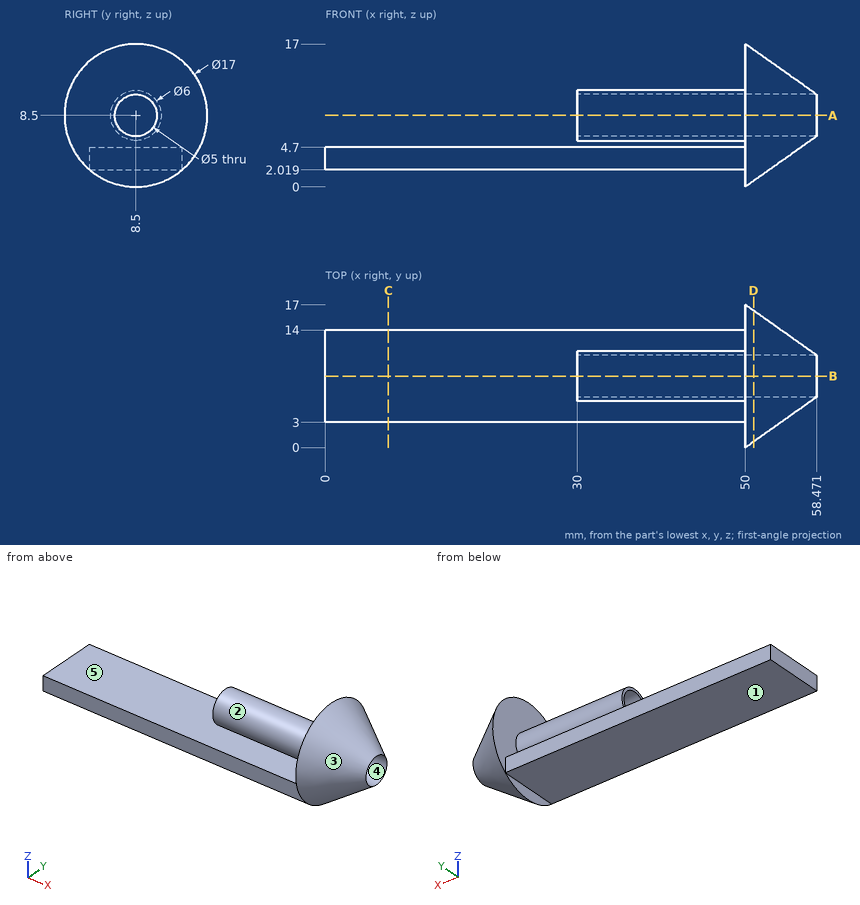
For this review, use the dimensioned drawing (mm, ordinates from the lowest corner) and the shaded views. A direction names the side the tool comes from. Round coordinates to 2 decimals unless told otherwise and drop trailing zeros. Write each loop counter-clockwise with the first axis right and the second up, starting at its lowest first coordinate (ties: lowest second). Pieces come first, ordered by that corner, then holes. Notation, with made-up numbers: (-37, 53.5) -> (-6, 53.5) arc R19 cw to (-6, 77.5) -> close; hole circle Ø1 at (-32.5, 4.5). An arc over 180 degrees is marked (long way). Use one line per item in the form item = value.
Q1. Consider section C-C (x = 7.5). State the section outline as (y, z) points.
Resolved:
outline = (3, 2.02) -> (14, 2.02) -> (14, 4.7) -> (3, 4.7) -> close
Q2. Consider section D-D (x = 51). State the section outline as (y, z) points, then the cut area to 3 significant figures.
Resolved:
outline = circle Ø15.58 at (8.5, 8.5); hole circle Ø5 at (8.5, 8.5)
area = 171 mm²
Q3. To check wall thickness, follow probe 1 along Z at (x, y) = (46.5, 8.5); probe 2 along Z at (x, y) = (11, 13.5); probe 3 along Z at (x, y) = (51.5, 8.5). State the ranges of each line that lie inside material, in increasing order. Write a range as from..to.
Resolved:
probe_1 = 2.02..4.7, 5.5..6, 11..11.5
probe_2 = 2.02..4.7
probe_3 = 1.06..6, 11..15.94
Q4. Machinability: for the marked faces 4 and 5, which of the approach directions +Z, -Z, +X, -X, +Y, -Y give a long, thin tool a straight path to every point of the face, cutting with its end or side? Answer none if there is none.
Resolved:
face_4 = +X, -X
face_5 = -X, +Y, -Y
Q5. The part is to be moulded in two halves that separate along Z. For the marked faces 1, 2 and 3, say which applies: released by +Z, released by -Z, zero draft, split by the parting line, or undercut.
Resolved:
face_1 = released by -Z
face_2 = undercut
face_3 = split by the parting line
Q6. Consider section B-B (y = 8.5). State the section outline as (x, z) points.
Resolved:
outline = (0, 2.02) -> (50, 2.02) -> (50, 0) -> (58.47, 6) -> (30, 6) -> (30, 5.5) -> (50, 5.5) -> (50, 4.7) -> (0, 4.7) -> close; (30, 11) -> (58.47, 11) -> (50, 17) -> (50, 11.5) -> (30, 11.5) -> close
Q7. Consider section A-A (z = 8.5). State the section outline as (x, y) points.
Resolved:
outline = (30, 5.5) -> (50, 5.5) -> (50, 0) -> (58.47, 6) -> (30, 6) -> close; (30, 11) -> (58.47, 11) -> (50, 17) -> (50, 11.5) -> (30, 11.5) -> close
Q8. Clearance check with flat-ended pins moving along their axes: pin 1 Ø0.8 at (x, z) = (29, 3.5) entering from -Y; pin 2 Ø4 at (x, y) = (30.5, 4) entering from +Z; pin 3 Ø8 at (x, y) = (15, 3) entering from -Z. State where each tip first meets the part, or that it passes through.
Resolved:
pin_1 = 3
pin_2 = 10.16
pin_3 = 2.02
